from build123d import *

# Parameters (mm, degrees)
EXTRUDE_1_DEPTH     = 3
CUT_EXTRUDE_1_DEPTH = 159.142340946


with BuildPart() as part:
    # Model → 凸台-拉伸1 (new body)
    with BuildSketch(Plane.XY):
        Polygon((92, 47), (92, 42), (89, 42), (89, 36), (92, 36), (92, 31), (98.5, 31), (98.5, 28), (104.5, 28), (104.5, 31), (110.5, 31), (110.5, 28), (116.5, 28), (116.5, 31), (122.5, 31), (122.5, 28), (128.5, 28), (128.5, 31), (134.5, 31), (134.5, 28), (140.5, 28), (140.5, 31), (146.5, 31), (147, 31), (147, 36), (150, 36), (150, 42), (147, 42), (147, 47), (140.5, 47), (140.5, 50), (134.5, 50), (134.5, 47), (128.5, 47), (128.5, 50), (122.5, 50), (122.5, 47), (116.5, 47), (116.5, 50), (110.5, 50), (110.5, 47), (104.5, 47), (104.5, 50), (98.5, 50), (98.5, 47), (92.5, 47), align=None)
    extrude(amount=EXTRUDE_1_DEPTH)

    # 草图2 → 切除-拉伸1 (cut, through all)
    with BuildSketch(Plane.XY.offset(3)):
        Polygon((133.622004458, 45.75), (133.622004458, 46.45), (134.322004458, 46.45), (142.322004458, 46.45), (143.022004458, 46.45), (143.022004458, 45.75), (143.022004458, 35.05), (133.622004458, 35.05), align=None)
        Polygon((114.197004458, 35.48), (101.757004458, 35.48), (101.757004458, 45.74), (101.757004458, 46.5), (114.197004458, 46.5), (114.197004458, 45.74), align=None)
    extrude(amount=-CUT_EXTRUDE_1_DEPTH, mode=Mode.SUBTRACT)


solid = part.part
Input: part model. Units: mm. Frame: model coordinates. A direction names the side the tool comes from. Give positions to 0.01 mm unless a question says otherwise; leave off trailing zeros. Order: outer loops, then holes, each group sorted by start corner. A loop starts at its lowest first (then second) coordinate and runs counter-clockwise, first axis right, second up. Notation, with made-up numbers: (88.5, 41) - (139.5, 41) arc R22 ccw to (139.5, 54) - close; hole circle Ø6 at (30, 77). An arc over 180 degrees is marked (long way). Answer as a JSON object with one key per item and string values. Group by question number.
Q1. Cut plane A-A, the plane y = 43.25. Output: boundary loops of the cut face in (x, z).
Q2. Mould query, pull axis X, two halves, no side actions, for faces 1 (the face through (147, 44, 1)), 2 (the face through (122.5, 30, 1)), 3 (the face through (122.5, 49, 1)), 4 (the face through (148, 36, 1)). Classes: pulls with the +X half, pulls with the -X half, needs draft (parallel to the pull), parting line crosses it, or undercut.
Q3. First-contact query: pin 1 Ø1.5 at (x, z) = (90.5, 2) entering from +Y; pin 2 Ø0.9 at (x, z) = (96, 2) entering from +Y; pin 3 Ø0.9 at (y, z) = (29, 1) entering from -X. Flat tips, straight axial feed; report the tip coordinate or a pass-through.
Q4. Set-up query: faces 5 (the face through (138, 46.45, 2)), 6 (the face through (144, 31, 1)), 7 (the face through (110.5, 49, 1)), 8 (the face through (95, 47, 1)). Return all of +Z, -Z, +X, -X, +Y, -Y with unobstructed straight access to the full face (end or side cutting, diameter ignored); none if empty.
Q5. Line query: probe 1 along X at (y, z) = (43.25, 1.9); probe 2 along X at (y, z) = (36.5, 2.8); probe 3 along X at (y, z) = (29, 2.45). Output: solid intervals per line, ascending.
Q6. Cut plane D-D, the plane y = 36.75. Output: boundary loops of the cut face in (x, z).
Q7. Cut plane B-B, the plane x = 112. Output: boundary loops of the cut face in (y, z).
Q8. Cut plane C-C, the plane z = 2.3. Count the separate pieces of the cut face and the enclosed holes in it, then the cut area to 3 significant figures.
Results:
{
 "1": {"outline": "(92, 0) - (101.76, 0) - (101.76, 3) - (92, 3) - close; (114.2, 0) - (133.62, 0) - (133.62, 3) - (114.2, 3) - close; (143.02, 0) - (147, 0) - (147, 3) - (143.02, 3) - close"},
 "2": {"face 1": "pulls with the +X half", "face 2": "undercut", "face 3": "undercut", "face 4": "needs draft"},
 "3": {"pin 1": "y = 42", "pin 2": "y = 47", "pin 3": "x = 98.5"},
 "4": {"face 5": "+Z, -Z", "face 6": "+Z, -Z, +X, -Y", "face 7": "+Z, -Z, +Y", "face 8": "+Z, -Z, -X, +Y"},
 "5": {"probe 1": "92 to 101.76, 114.2 to 133.62, 143.02 to 147", "probe 2": "89 to 101.76, 114.2 to 133.62, 143.02 to 150", "probe 3": "98.5 to 104.5, 110.5 to 116.5, 122.5 to 128.5, 134.5 to 140.5"},
 "6": {"outline": "(89, 0) - (101.76, 0) - (101.76, 3) - (89, 3) - close; (114.2, 0) - (133.62, 0) - (133.62, 3) - (114.2, 3) - close; (143.02, 0) - (150, 0) - (150, 3) - (143.02, 3) - close"},
 "7": {"outline": "(28, 0) - (35.48, 0) - (35.48, 3) - (28, 3) - close; (46.5, 0) - (50, 0) - (50, 3) - (46.5, 3) - close"},
 "8": {"separate pieces": "1", "enclosed holes": "2", "area": "816 mm^2"}
}
